Could you check a few things on this model? Use its own coordinates, in mm. A direction names the side the tool comes from. Coordinates: 2 decimals unless noted, no trailing zeros. Write each loop counter-clockwise with the first axis right and the second up, starting at its lowest first coordinate (ties: lowest second). Pieces come first, ordered by that corner, then holes.
Autodesk Inventor part; units mm, degrees
ref_plane "YZ Plane" through (0, 0, 0) normal (1, 0, 0) x (0, 1, 0)
ref_plane "XZ Plane" through (0, 0, 0) normal (0, 1, 0) x (-1, 0, 0)
ref_plane "XY Plane" through (0, 0, 0) normal (0, 0, 1) x (1, 0, 0)
sketch "Sketch1" plane through (0, 0, 0) normal (0, 1, 0) x (-1, 0, 0)
  line L0 (46, 0) -> (-35, 0) construction
  line L1 (0, 54.3949) -> (0, -60) construction
  line L2 (10, 20) -> (-10, 20)
  line L3 (-10, 20) -> (-10, -20)
  line L4 (-10, -20) -> (10, -20)
  line L5 (10, -20) -> (10, 20)
  line L6 (17, -28) -> (17, 28)
  circle A0 centre (5, 24.25) radius 0.5
  circle A1 centre (-5, 24.25) radius 0.5
  line L7 (14.6784, 24.25) -> (-18, 24.25) construction
  circle A2 centre (5, -24.25) radius 0.5
  circle A3 centre (-5, -24.25) radius 0.5
  circle A4 centre (13.5, -18.75) radius 1.5
  line L8 (-17, 28) -> (-17, -28)
  line L9 (17, -28) -> (-17, -28)
  line L10 (17, 28) -> (33.782, 48)
  line L11 (17, 28) -> (43.1081, 28) construction
  line L12 (-17, 28) -> (-33.782, 48)
  arc A5 (33.782, 48) -> (-33.782, 48) centre (0, -24.5174) ccw
  line L13 (20, 48) -> (-20, 48)
  line L14 (-20, 48) -> (-20, 45)
  line L15 (-20, 45) -> (20, 45)
  line L16 (20, 45) -> (20, 48)
  circle A6 centre (0, 35) radius 1.5
  circle A7 centre (-13.5, -18.75) radius 1.5
  point P0 (0, 0)
  dimension "d0" = 40
  dimension "d1" = 20
  dimension "d2" = 7
  dimension "d6" = 20
  dimension "d7" = 10
  dimension "d11" = 1
  dimension "d12" = 1
  dimension "d13" = 5
  dimension "d14" = 5
  dimension "d15" = 4.25
  dimension "d16" = 3
  dimension "d29" = 3.5
  dimension "d34" = 8
  dimension "d35" = 50
  dimension "d36" = 20
  dimension "d37" = 56
  dimension "d38" = 80
  dimension "d39" = 40
  dimension "d41" = 3
  dimension "d42" = 25
  dimension "d43" = 9.25
  dimension "d44" = 3
  dimension "d45" = 10
extrude "Extrusion2" add sketch "Sketch1" along normal blind 3
fillet "Fillet2" radius 2 6 edges at (33.782, 1.5, 48) (-33.782, 1.5, 48) (17, 1.5, 28) (-17, 1.5, 28) (-17, 1.5, -28) (17, 1.5, -28)
properties part number "bracket_camera_top"
1. Please list where these lines run through material, in increasing order: line 1 along Z through (x, y) = (0, 0.6); line 2 along X through (y, z) = (2.65, 0.5); line 3 along Z through (x, y) = (12.5, 2.1).
Verdict:
line 1: z = -28 to -20, 20 to 33.5, 36.5 to 45, 48 to 55.48
line 2: x = -17 to -10, 10 to 17
line 3: z = -28 to -19.87, -17.63 to 45, 48 to 54.5
2. I want a section at B-B on x = 0. Please give me the cut outline in (y, z), plus the area to 3 significant figures.
Verdict:
outline: (0, -28) - (3, -28) - (3, -20) - (0, -20) - close; (0, 20) - (3, 20) - (3, 33.5) - (0, 33.5) - close; (0, 36.5) - (3, 36.5) - (3, 45) - (0, 45) - close; (0, 48) - (3, 48) - (3, 55.48) - (0, 55.48) - close
area: 112 mm2
3. For pin 1 (0.9 mm diameter, centred on y = 1.5, z = 46, fed in from -X); pin 2 (1.5 mm diameter, centred on x = 3, y = 1, fed in from +Z); pin 3 (0.9 mm diameter, centred on y = 1.5, z = 11.5, fed in from -X); pin 4 (2.5 mm diameter, centred on x = -13.5, z = -18.75, fed in from -Y), each with a flat end and sliding along its axis, tell me the tip position at first contact or that it passes through.
Verdict:
pin 1: stops at x = -32.38
pin 2: stops at z = 55.45
pin 3: stops at x = -17
pin 4: passes through
4. I want a section at C-C on y = 2.45. Give the number of separate pieces and of enclosed holes in the cut face, plus the area to 3 significant figures.
Verdict:
separate pieces: 1
enclosed holes: 9
area: 2,310 mm2
5. On a 3-axis mill with a long thin cutter (end or side, diameter ignored), from which of +Z, -Z, +X, -X, +Y, -Y can I reach the whole of each face in a straight line? I mean faces 5 (the face through (32.483, 1.521, 47.745)), 6 (the face through (-10, 1, 0)), 7 (the face through (-17, 1, 0)). Say none if no direction works.
Verdict:
face 5: +X, +Y, -Y
face 6: +Y, -Y
face 7: -Z, -X, +Y, -Y
6. If we mould it in two halves opening along X, with no side actions, what happens to faces 1 (the face through (16.43, 1.52, -27.4)), 2 (the face through (0.45, 1.48, 55.48)), 3 (the face through (20, 1, 47)), 4 (the face through (0, 1, 48))? For each: pulls with the +X half, pulls with the -X half, needs draft (parallel to the pull), parting line crosses it, or undercut.
Verdict:
face 1: pulls with the +X half
face 2: parting line crosses it
face 3: undercut
face 4: undercut
7. I want a section at A-A on z = -18.75. Please give me the cut outline in (x, y).
Verdict:
outline: (-17, 0) - (-15, 0) - (-15, 3) - (-17, 3) - close; (-12, 0) - (-10, 0) - (-10, 3) - (-12, 3) - close; (10, 0) - (12, 0) - (12, 3) - (10, 3) - close; (15, 0) - (17, 0) - (17, 3) - (15, 3) - close
8. I want a section at D-D on z = 6. Please give me the cut outline in (x, y), plus the area to 3 significant figures.
Verdict:
outline: (-17, 0) - (-10, 0) - (-10, 3) - (-17, 3) - close; (10, 0) - (17, 0) - (17, 3) - (10, 3) - close
area: 42.0 mm2
